Source: CAD feature listing. Evaluate the final solid. Frame: model axes, mm. A direction names the side the tool comes from. Round coordinates to 2 decimals unless told otherwise and drop trailing zeros. Write each loop counter-clockwise with the first axis right and the second up, starting at its lowest first coordinate (ties: lowest second). Pieces come first, ordered by that corner, then holes. Notation, with made-up numbers: M 59,88.25 L 74,88.25 A25 ccw 74,101.25 Z; hole C 19,80.25 d1. An arc over 180 degrees is marked long. Use a Markdown table: item, result.
```python
from build123d import *

# Parameters (mm, degrees)
SKETCH3_W        = 4
SKETCH3_H        = 3
WASHER_START     = 140
SKETCH4_R        = 32
WASHER_DEPTH     = 6
CRANK_START      = 146
CRANK_BOLT_DEPTH = 10


with BuildPart() as part:
    # Sketch1 → Balancer (revolve)
    with BuildSketch(Plane(origin=(0, 0, 0), x_dir=(0, 0, -1), z_dir=(1, 0, 0)), mode=Mode.PRIVATE) as balancer_sk:
        with BuildLine():
            Line((-98, 25.05), (-98, 98.5))
            ThreePointArc((-98, 98.5), (-98.439339828, 99.560660172), (-99.5, 100))
            Line((-99.5, 100), (-114.5, 100))
            ThreePointArc((-114.5, 100), (-115.560660172, 99.560660172), (-116, 98.5))
            Line((-116, 98.5), (-116, 94))
            Line((-116, 94), (-138.5, 94))
            ThreePointArc((-138.5, 94), (-139.560660172, 93.560660172), (-140, 92.5))
            Line((-140, 92.5), (-140, 25.05))
            Line((-140, 25.05), (-98, 25.05))
        make_face()
    revolve(balancer_sk.sketch.rotate(Axis((0, 0, 80), (0, 0, 1)), 90), axis=Axis((0, 0, 80), (0, 0, 1)))

    # Sketch2 → Belt Grooves (revolve, cut)
    with BuildSketch(Plane(origin=(0, 0, 0), x_dir=(0, 0, -1), z_dir=(1, 0, 0)), mode=Mode.PRIVATE) as belt_grooves_sk:
        Polygon((-119, 96), (-120.5, 91.5), (-122, 96), align=None)
        Polygon((-122.4, 96), (-123.9, 91.5), (-125.4, 96), align=None)
        Polygon((-125.8, 96), (-127.3, 91.5), (-128.8, 96), align=None)
        Polygon((-129.2, 96), (-130.7, 91.5), (-132.2, 96), align=None)
        Polygon((-132.6, 96), (-134.1, 91.5), (-135.6, 96), align=None)
        Polygon((-136, 96), (-137.5, 91.5), (-139, 96), align=None)
    revolve(belt_grooves_sk.sketch.rotate(Axis((0, 0, 80), (0, 0, 1)), 90), axis=Axis((0, 0, 80), (0, 0, 1)), mode=Mode.SUBTRACT)

    # Sketch3 → Isolator Groove (revolve, cut)
    with BuildSketch(Plane(origin=(0, 0, 0), x_dir=(0, 0, -1), z_dir=(1, 0, 0)), mode=Mode.PRIVATE) as isolator_groove_sk:
        with Locations((-139, 65.5)):
            Rectangle(SKETCH3_W, SKETCH3_H)
    revolve(isolator_groove_sk.sketch.rotate(Axis((0, 0, 80), (0, 0, 1)), 90), axis=Axis((0, 0, 80), (0, 0, 1)), mode=Mode.SUBTRACT)

    # Sketch4 → Washer (add)
    with BuildSketch(Plane.XY.offset(WASHER_START)):
        Circle(SKETCH4_R)
    extrude(amount=WASHER_DEPTH)

    # Sketch5 → Crank Bolt (add)
    with BuildSketch(Plane.XY.offset(CRANK_START)):
        Polygon((16, 0), (8, 13.856406461), (-8, 13.856406461), (-16, 0), (-8, -13.856406461), (8, -13.856406461), align=None)
    extrude(amount=CRANK_BOLT_DEPTH)


solid = part.part
```
Q1. Section A-A on z = 150.5. Return loops of the section in (x, y), plus the area to 3 significant figures.
Results are:
| item | result |
|---|---|
| outline | M -16,0 L -8,-13.86 L 8,-13.86 L 16,0 L 8,13.86 L -8,13.86 Z |
| area | 665 mm^2 |
Q2. First-contact query: pin 1 Ø1 at (x, z) = (33, 111.5) entering from +Y; pin 2 Ø12 at (x, z) = (75.5, 142.5) entering from -Y; pin 3 Ø25 at (x, y) = (-4.5, 0) entering from -Z. Flat tips, straight axial feed; report the tip coordinate or a pass-through.
Results are:
| item | result |
|---|---|
| pin 1 | y = 94.57 |
| pin 2 | y = -61.93 |
| pin 3 | z = 140 |
Q3. Section B-B on z = 106.5. Return loops of the section in (x, y).
Results are:
| item | result |
|---|---|
| outline | C 0,0 d200; hole C 0,0 d50.1 |
Q4. Reachability of faces 1 (the flat face through (-11.94, 7.03, 150.93)), 2 (the flat face through (0, 13.856, 151)), 3 (the flat face through (-12.056, -6.831, 150.93)), 4 (the flat face through (54.3, 34.4, 137)) from +Z, -Z, +X, -X, +Y, -Y: full face, straight path, thin tool, end or side. Return the list, or none.
Results are:
| item | result |
|---|---|
| face 1 | +Z, -X, +Y |
| face 2 | +Z, +X, -X, +Y |
| face 3 | +Z, -X, -Y |
| face 4 | +Z |
Q5. Line query: L1, parallel to Y at x = 0, z = 118; L2, parallel to Z at x = -75, y = 21.5; L3, parallel to Z at x = 19.5, y = 6. Output: solid intervals per line, ascending.
Results are:
| item | result |
|---|---|
| L1 | -94 to -25.05, 25.05 to 94 |
| L2 | 98 to 140 |
| L3 | 140 to 146 |
Q6. Mould query, pull axis Y, two halves, no side actions, for faces 5 (the cylindrical face through (-30.92, 59.44, 138.48)), 6 (the cylindrical face through (12.24, -93.2, 132.41)), 7 (the flat face through (0, 0, 156)). Classes: +Y half, -Y half, draft (parallel to the pull), parting line (faces both ways), or undercut.
Results are:
| item | result |
|---|---|
| face 5 | undercut |
| face 6 | parting line |
| face 7 | draft |
